```python
from build123d import *

# Parameters (mm, degrees)
SKETCH_1_R          = 1
SKETCH_1_R_2        = 5
EXTRUDE_1_DEPTH     = 2
SKETCH_2_R          = 7
EXTRUDE_2_DEPTH     = 16
EXTRUDE_2_DRAFT     = -45
SKETCH_3_R          = 5
CUT_EXTRUDE_1_DEPTH = 37.249137921
CUT_EXTRUDE_1_DRAFT = 45
EXTRUDE_3_REACH     = 38.249
EXTRUDE_5_REACH     = 38.249
SKETCH_5_R          = 1


with BuildPart() as part:
    # Эскиз1 → Бобышка-Вытянуть1 (new body)
    with BuildSketch(Plane.XY):
        with BuildLine():
            ThreePointArc((-1.4494714, 6.848286841), (-7, 0), (-1.4494714, -6.848286841))
            ThreePointArc((-1.4494714, -6.848286841), (2.194861582, -9.218418644), (4.380086565, -5.46029685))
            ThreePointArc((4.380086565, -5.46029685), (7, 0), (4.380086565, 5.46029685))
            ThreePointArc((4.380086565, 5.46029685), (2.194861582, 9.218418644), (-1.4494714, 6.848286841))
        make_face()
        with Locations((1.5, 6.3)):
            Circle(SKETCH_1_R, mode=Mode.SUBTRACT)
        with Locations((1.5, -6.3)):
            Circle(SKETCH_1_R, mode=Mode.SUBTRACT)
        Circle(SKETCH_1_R_2, mode=Mode.SUBTRACT)
    extrude(amount=EXTRUDE_1_DEPTH)


with BuildPart() as extrude_2_tool:
    # Эскиз2 → Бобышка-Вытянуть2 (with draft: the straight prism first)
    with BuildSketch(Plane(origin=(0, 0, 0), x_dir=(-1, 0, 0), z_dir=(0, 0, -1))):
        Circle(SKETCH_2_R)
    extrude(amount=EXTRUDE_2_DEPTH)
    # Бобышка-Вытянуть2: the draft: its side faces are tilted about the plane it starts from
    extrude_2_sides = [extrude_2_tool.faces().sort_by_distance(p)[0] for p in [
        (7, 0, -8),
    ]]
    draft(extrude_2_sides, Plane(origin=(0, 0, 0), x_dir=(-1, 0, 0), z_dir=(0, 0, -1)), EXTRUDE_2_DRAFT)


with BuildPart() as part_1:
    add(part.part)

    # Бобышка-Вытянуть2: add extrude_2_tool
    add(extrude_2_tool.part)


with BuildPart() as cut_extrude_1_tool:
    # Эскиз3 → Вырез-Вытянуть1 (with draft: the straight prism first)
    with BuildSketch(Plane.XY):
        Circle(SKETCH_3_R)
    extrude(amount=-CUT_EXTRUDE_1_DEPTH)
    # Вырез-Вытянуть1: the draft: its side faces are tilted about the plane it starts from
    cut_extrude_1_sides = [cut_extrude_1_tool.faces().sort_by_distance(p)[0] for p in [
        (-5, 0, -18.62456896),
    ]]
    draft(cut_extrude_1_sides, Plane.XY, CUT_EXTRUDE_1_DRAFT)


with BuildPart() as part_2:
    add(part_1.part)

    # Вырез-Вытянуть1: cut by cut_extrude_1_tool
    add(cut_extrude_1_tool.part, mode=Mode.SUBTRACT)

    # Эскиз4 → Бобышка-Вытянуть3 (add, up to next)
    with BuildSketch(Plane(origin=(0, 0, 0), x_dir=(-1, 0, 0), z_dir=(0, 0, -1)), mode=Mode.PRIVATE) as extrude_3_sk1:
        with BuildLine():
            ThreePointArc((-4.380086565, -5.46029685), (-3.467221669, -6.080984616), (-2.468130818, -6.550445043))
            ThreePointArc((-2.468130818, -6.550445043), (-1.731620527, -7.272806215), (-0.74860738, -6.959855386))
            ThreePointArc((-0.74860738, -6.959855386), (0.354844302, -6.991000323), (1.4494714, -6.848286841))
            ThreePointArc((1.4494714, -6.848286841), (-2.194861582, -9.218418644), (-4.380086565, -5.46029685))
        make_face()
    extrude_3_tool1 = extrude(extrude_3_sk1.sketch, amount=EXTRUDE_3_REACH, mode=Mode.PRIVATE) - part_2.part
    # Эскиз4 → Бобышка-Вытянуть3 (add, up to next)
    with BuildSketch(Plane(origin=(0, 0, 0), x_dir=(-1, 0, 0), z_dir=(0, 0, -1)), mode=Mode.PRIVATE) as extrude_3_sk2:
        with BuildLine():
            ThreePointArc((1.4494714, 6.848286841), (0.354844302, 6.991000323), (-0.74860738, 6.959855386))
            ThreePointArc((-0.74860738, 6.959855386), (-1.731620527, 7.272806215), (-2.468130818, 6.550445043))
            ThreePointArc((-2.468130818, 6.550445043), (-3.467221669, 6.080984616), (-4.380086565, 5.46029685))
            ThreePointArc((-4.380086565, 5.46029685), (-2.194861582, 9.218418644), (1.4494714, 6.848286841))
        make_face()
    extrude_3_tool2 = extrude(extrude_3_sk2.sketch, amount=EXTRUDE_3_REACH, mode=Mode.PRIVATE) - part_2.part
    add(extrude_3_tool1.solids().sort_by_distance((1.839664, -7.72659, 0))[0])
    add(extrude_3_tool2.solids().sort_by_distance((1.839664, 7.72659, 0))[0])

    # Эскиз5 → Бобышка-Вытянуть5 (add, up to next)
    with BuildSketch(Plane.XY, mode=Mode.PRIVATE) as extrude_5_sk1:
        with Locations((1.5, 6.3)):
            Circle(SKETCH_5_R)
    extrude_5_tool1 = extrude(extrude_5_sk1.sketch, amount=-EXTRUDE_5_REACH, mode=Mode.PRIVATE) - part_2.part
    # Эскиз5 → Бобышка-Вытянуть5 (add, up to next)
    with BuildSketch(Plane.XY, mode=Mode.PRIVATE) as extrude_5_sk2:
        with Locations((1.5, -6.3)):
            Circle(SKETCH_5_R)
    extrude_5_tool2 = extrude(extrude_5_sk2.sketch, amount=-EXTRUDE_5_REACH, mode=Mode.PRIVATE) - part_2.part
    add(extrude_5_tool1.solids().sort_by_distance((1.5, 6.3, 0))[0])
    add(extrude_5_tool2.solids().sort_by_distance((1.5, -6.3, 0))[0])


solid = part_2.part
```
Input: part model. Units: mm. Frame: model coordinates. A direction names the side the tool comes from. Coordinates: 2 decimals unless noted, no trailing zeros. Loops run counter-clockwise (first coordinate to the right, second up) from the corner with the lowest first, then second, coordinate; pieces in that order, holes last. Notation, with made-up numbers: M 2.5,66.5 L 20.5,66.5 A17 ccw 20.5,74.5 Z; hole C 53.5,-13.5 d11. An arc over 180 degrees is marked long. Use a Markdown table: item, result. Add a question column.
1) Section A-A, the plane y = 0. Return the cut outline in (x, z).
2) Line query: L1, parallel to Y at x = 1.5, z = 1.55; L2, parallel to X at y = -11, z = -12.25; L3, parallel to Y at x = -8.5, z = -10.5. Output: solid intervals per line, ascending. Write a range as from..to.
3) Section B-B, the plane z = -5.25. Return the cut outline in (x, y).
4) Set-up query: faces 1 (the cylindrical face through (-7, 0, 1)), 2 (the cylindrical face through (7, 0, 1)), 3 (the flat face through (5, 2, 2)), 4 (the cylindrical face through (1.283, -7.276, 0.986)). Return all of +Z, -Z, +X, -X, +Y, -Y with unobstructed straight access to the full face (end or side cutting, diameter ignored); none if empty.
5) Pin query (flat end, axial travel): P1, Ø6, axis at x = 13, z = -0.5, coming from the -Y side; P2, Ø1.8, axis at x = 1.5, y = 6.3, coming from the +Z side; P3, Ø3, axis at x = 1.5, y = -6.3, coming from the +Z side; P4, Ø4, axis at x = -10, z = -8, coming from the +Y side. Return the tip coordinate at first contact, or that it passes through.
Answer below:
| question | item | result |
|---|---|---|
| 1 | outline | M -23,-16 L -21,-16 L -5,0 L -5,2 L -7,2 L -7,0 Z; M 5,0 L 21,-16 L 23,-16 L 7,0 L 7,2 L 5,2 Z |
| 2 | L1 | -9.3..-7.3, -5.3..-4.77, 4.77..5.3, 7.3..9.3 |
| 2 | L2 | -15.8..-13.29, 13.29..15.8 |
| 2 | L3 | -15.3..-12.96, 12.96..15.3 |
| 3 | outline | C 0,0 d24.5; hole C 0,0 d20.5 |
| 4 | face 1 | +Z, -X |
| 4 | face 2 | +Z, +X |
| 4 | face 3 | +Z, +X, -X, +Y, -Y |
| 4 | face 4 | +Z |
| 5 | P1 | through |
| 5 | P2 | z = 0 |
| 5 | P3 | z = 2 |
| 5 | P4 | y = 14.11 |
